```python
from build123d import *

# Parameters (mm, degrees)
F1_DEPTH = 3.885
F2_R     = 2.385
F3_DEPTH = 12.5
F4_R     = 3.8627416998


with BuildPart() as f1:
    # F0 (on Front) → F1 (new body, symmetric)
    with BuildSketch(Plane.XZ):
        with BuildLine():
            ThreePointArc((-3.675, 0), (0, -3.675), (3.675, 0))
            ThreePointArc((3.675, 0), (0, 3.675), (-3.675, 0))
        make_face()
        with BuildLine():
            ThreePointArc((2.375, 0.1541914395), (2.3787496716, 0.0771362431), (2.38, 0))
            ThreePointArc((2.38, 0), (2.3787496716, -0.0771362431), (2.375, -0.1541914395))
            Line((2.375, -0.1541914395), (2.375, -0.89))
            Line((2.375, -0.89), (2.2073287023, -0.89))
            ThreePointArc((2.2073287023, -0.89), (1.6829141392, -1.6829141392), (0.89, -2.2073287023))
            Line((0.89, -2.2073287023), (0.89, -2.375))
            Line((0.89, -2.375), (0.1541914395, -2.375))
            ThreePointArc((0.1541914395, -2.375), (0, -2.38), (-0.1541914395, -2.375))
            Line((-0.1541914395, -2.375), (-0.89, -2.375))
            Line((-0.89, -2.375), (-0.89, -2.2073287023))
            ThreePointArc((-0.89, -2.2073287023), (-1.6829141392, -1.6829141392), (-2.2073287023, -0.89))
            Line((-2.2073287023, -0.89), (-2.375, -0.89))
            Line((-2.375, -0.89), (-2.375, -0.1541914395))
            ThreePointArc((-2.375, -0.1541914395), (-2.38, 0), (-2.375, 0.1541914395))
            Line((-2.375, 0.1541914395), (-2.375, 0.89))
            Line((-2.375, 0.89), (-2.2073287023, 0.89))
            ThreePointArc((-2.2073287023, 0.89), (-1.6829141392, 1.6829141392), (-0.89, 2.2073287023))
            Line((-0.89, 2.2073287023), (-0.89, 2.375))
            Line((-0.89, 2.375), (-0.1541914395, 2.375))
            ThreePointArc((-0.1541914395, 2.375), (0, 2.38), (0.1541914395, 2.375))
            Line((0.1541914395, 2.375), (0.89, 2.375))
            Line((0.89, 2.375), (0.89, 2.2073287023))
            ThreePointArc((0.89, 2.2073287023), (1.6829141392, 1.6829141392), (2.2073287023, 0.89))
            Line((2.2073287023, 0.89), (2.375, 0.89))
            Line((2.375, 0.89), (2.375, 0.1541914395))
        make_face(mode=Mode.SUBTRACT)
        with BuildLine():
            Line((3.675, -11.2), (3.675, 0))
            ThreePointArc((3.675, 0), (0, -3.675), (-3.675, 0))
            Line((-3.675, 0), (-3.675, -11.2))
            Line((-3.675, -11.2), (3.675, -11.2))
        make_face()
        with BuildLine():
            Line((-0.89, -2.2073287023), (-0.89, -0.89))
            Line((-0.89, -0.89), (-2.2073287023, -0.89))
            ThreePointArc((-2.2073287023, -0.89), (-1.6829141392, -1.6829141392), (-0.89, -2.2073287023))
        make_face()
        with BuildLine():
            Line((-2.2073287023, 0.89), (-0.89, 0.89))
            Line((-0.89, 0.89), (-0.89, 2.2073287023))
            ThreePointArc((-0.89, 2.2073287023), (-1.6829141392, 1.6829141392), (-2.2073287023, 0.89))
        make_face()
        with BuildLine():
            Line((0.89, 0.89), (2.2073287023, 0.89))
            ThreePointArc((2.2073287023, 0.89), (1.6829141392, 1.6829141392), (0.89, 2.2073287023))
            Line((0.89, 2.2073287023), (0.89, 0.89))
        make_face()
        with BuildLine():
            ThreePointArc((0.89, -2.2073287023), (1.6829141392, -1.6829141392), (2.2073287023, -0.89))
            Line((2.2073287023, -0.89), (0.89, -0.89))
            Line((0.89, -0.89), (0.89, -2.2073287023))
        make_face()
    extrude(amount=F1_DEPTH, both=True)

    # F2 (on face) → F3 (cut, symmetric)
    with BuildSketch(Plane.YZ.offset(3.675)):
        with Locations((0, -7.505)):
            Circle(F2_R)
    extrude(amount=F3_DEPTH, both=True, mode=Mode.SUBTRACT)

    # F4
    f4_edges = [f1.edges().sort_by_distance(p)[0] for p in [
        (0, 3.885, -11.2),
        (0, -3.885, -11.2),
    ]]
    fillet(f4_edges, radius=F4_R)


solid = f1.part
```
Source: CAD feature listing. Evaluate the final solid. Frame: model axes, mm. A direction names the side the tool comes from. Give positions to 0.01 mm unless a question says otherwise; leave off trailing zeros. Order: outer loops, then holes, each group sorted by start corner. A loop starts at its lowest first (then second) coordinate and runs counter-clockwise, first axis right, second up.
(1) Section query C-C (z = -7). Return the cut outline in (x, y) (3 decimals), plus the area to 3 significant figures.
(2) Contact query for flat-ended pins moving along their axis: P1, Ø4, axis at y = -3, z = 2, coming from the +X side (3 decimals); P2, Ø1.6, axis at y = -1, z = 2, coming from the +X side; P3, Ø0.6, axis at y = -0.5, z = 0.5, coming from the -X side; P4, Ø1.2, axis at x = 1.5, y = -1.5, coming from the -Z side. Output: stop coordinate, or through.
(3) Section query A-A (y = -0.5). Return the cut outline in (x, z) (3 decimals).
(4) Material intervals for line 1 along X through (y, z) = (3.75, -0.25) (3 decimals); line 2 along Z through (x, y) = (1.25, 0); line 3 along Z through (x, y) = (-2, 0), sorted ascending.
(5) Section query B-B (x = -0.5). Return the cut outline in (y, z) (3 decimals), plus the area to 3 significant figures.
(6) Access query for faces 5 (the face through (-2, 0, 0.89)), 6 (the face through (0.05, -2.78, -10.04)). Directions: +Z, -Z, +X, -X, +Y, -Y. A direction counts if a zero-diameter tool reaches every point of the face in a straight line with its end or side. Return the directions, or none.
(7) Section query D-D (y = -2.75). Return the cut outline in (x, z) (3 decimals), plus the area to 3 significant figures.
(8) Pull-direction query (Z, two-part tool) for faces 1 (the face through (0.05, -0.31, -5.14)), 2 (the face through (3.675, 0, -4)), 3 (the face through (2, 0, 0.89)), 4 (the face through (0.05, 2.78, -10.04)); classes: +Z half, -Z half, draft (parallel to the pull), parting line (faces both ways), or undercut.
Outcome:
1. outline: (-3.675, -3.885) - (3.675, -3.885) - (3.675, -2.331) - (-3.675, -2.331) - close; (-3.675, 2.331) - (3.675, 2.331) - (3.675, 3.885) - (-3.675, 3.885) - close
1. area: 22.8 mm2
2. P1: stops at x = 3.675
2. P2: stops at x = 3.47
2. P3: stops at x = -3.67
2. P4: stops at z = -11.1
3. outline: (-3.675, -11.17) - (3.675, -11.17) - (3.675, -9.837) - (-3.675, -9.837) - close; (-3.675, -5.173) - (3.675, -5.173) - (3.675, 0) arc R3.675 ccw to (-3.675, 0) - close; hole (-2.375, -0.89) - (-0.89, -0.89) - (-0.89, -2.375) - (-0.154, -2.375) arc R2.38 ccw to (0.154, -2.375) - (0.89, -2.375) - (0.89, -0.89) - (2.375, -0.89) - (2.375, -0.154) arc R2.38 ccw to (2.375, 0.154) - (2.375, 0.89) - (0.89, 0.89) - (0.89, 2.375) - (0.154, 2.375) arc R2.38 ccw to (-0.154, 2.375) - (-0.89, 2.375) - (-0.89, 0.89) - (-2.375, 0.89) - (-2.375, 0.154) arc R2.38 ccw to (-2.375, -0.154) - close
4. line 1: x = -3.675 to -2.375, 2.375 to 3.675
4. line 2: z = -11.2 to -9.89, -5.12 to -0.89, 0.89 to 3.46
4. line 3: z = -11.2 to -9.89, -5.12 to -0.89, 0.89 to 3.08
5. outline: (-3.885, -7.337) arc R3.863 ccw to (-0.022, -11.2) - (0.022, -11.2) arc R3.863 ccw to (3.885, -7.337) - (3.885, -2.375) - (-3.885, -2.375) - close; (-3.885, 2.375) - (3.885, 2.375) - (3.885, 3.641) - (-3.885, 3.641) - close; hole circle Ø4.77 at (0, -7.505)
5. area: 54.1 mm2
6. face 5: +Y, -Y
6. face 6: -Z, +X, -X, -Y
7. outline: (-3.675, -10.072) - (3.675, -10.072) - (3.675, 0) arc R3.675 ccw to (-3.675, 0) - close; hole (-2.375, -0.89) - (-0.89, -0.89) - (-0.89, -2.375) - (-0.154, -2.375) arc R2.38 ccw to (0.154, -2.375) - (0.89, -2.375) - (0.89, -0.89) - (2.375, -0.89) - (2.375, -0.154) arc R2.38 ccw to (2.375, 0.154) - (2.375, 0.89) - (0.89, 0.89) - (0.89, 2.375) - (0.154, 2.375) arc R2.38 ccw to (-0.154, 2.375) - (-0.89, 2.375) - (-0.89, 0.89) - (-2.375, 0.89) - (-2.375, 0.154) arc R2.38 ccw to (-2.375, -0.154) - close
7. area: 81.5 mm2
8. face 1: undercut
8. face 2: draft
8. face 3: undercut
8. face 4: -Z half
